Check sheet for the modelled part. Datum: model origin and axes. Units: mm. A direction names the side the tool comes from. Coordinates: 2 decimals unless noted, no trailing zeros. Write each loop counter-clockwise with the first axis right and the second up, starting at its lowest first coordinate (ties: lowest second). Pieces come first, ordered by that corner, then holes. Notation, with made-up numbers: (14, -25) -> (44, -25) arc R17 cw to (44, -21) -> close; hole circle Ø5 at (40, 38). An arc over 180 degrees is marked (long way). One line per item, written item: value. Start each with the question number.
1) Sectioned sample at D-D on x = -78. Enter the section's corners in (y, z), plus the area to 3 significant figures.
2) Sectioned sample at A-A on x = 0. Enter the section's corners in (y, z), plus the area to 3 significant figures.
3) Set-up check for faces 5 (the flat face through (29, -224, 7)), 6 (the flat face through (-82.516, -196.574, 3.451)): record each of +Z, -Z, +X, -X, +Y, -Y from which the full face is reachable in a straight line by a thin tool's end or side.
4) Gauge pin test, flat ends, axial feed: P1, Ø3, axis at x = -57, z = 4.5, coming from the -Y side; P2, Ø1.5, axis at x = 26.5, y = -417.5, coming from the -Z side; P3, Ø2, axis at x = -54.5, z = 4.5, coming from the +Y side; P4, Ø2, axis at x = -0.5, z = 1, coming from the -Y side. Record the tip position at first contact, or that the pin passes through.
5) Draft check along Y on faces 1 (the cylindrical face through (-178.984, -61.978, 3.451)), 2 (the flat face through (-100.6, 13.3, 3.5)), 3 (the cylindrical face through (-125.96, -269.94, 3.45)), 4 (the cylindrical face through (22.38, -43.028, 3.451)). Enter one of: +Y half, -Y half, draft (parallel to the pull), parting line (faces both ways), or undercut.
6) Sectioned sample at B-B on z = 5.75. Enter the section's corners in (x, y), plus the area to 3 significant figures.
7) Scan lines: line 1 along X through (y, z) = (-92, 2.25); line 2 along X through (y, z) = (-175, 4.75); line 3 along Y through (x, z) = (-134, 4). Record each from-to range of solid material in increasing order. Write a range as [from, to].
8) Sectioned sample at C-C on y = -117. Enter the section's corners in (x, z), plus the area to 3 significant figures.
```python
from build123d import *

# Parameters (mm, degrees)
SKETCH1_R      = 48.5
SKETCH1_R_2    = 46
EXTRUDE1_DEPTH = 7


with BuildPart() as part:
    # Sketch1 → Extrude1 (new body)
    with BuildSketch(Plane.XY):
        with BuildLine():
            Line((-181.296983893, -100.123158622), (-146.60541801, -252.204231237))
            ThreePointArc((-146.60541801, -252.204231237), (-125.550644715, -269.965422259), (-102.674010073, -254.621922903))
            Line((-102.674010073, -254.621922903), (-61.786520036, -136.878304089))
            ThreePointArc((-61.786520036, -136.878304089), (-17.984074435, -110.454979585), (15.979150749, -148.708680759))
            Line((15.979150749, -148.708680759), (22.803821631, -360))
            ThreePointArc((22.803821631, -360), (39.422409163, -464.1696592), (81.472905946, -560.912881546))
            Line((81.472905946, -560.912881546), (119.560838109, -625.042587939))
            ThreePointArc((119.560838109, -625.042587939), (124.22199896, -626.808768638), (126.985562325, -622.660451839))
            Line((126.985562325, -622.660451839), (122.910471509, -574.827683832))
            ThreePointArc((122.910471509, -574.827683832), (122.67212546, -573.014734487), (122.269195455, -571.231130949))
            Line((122.269195455, -571.231130949), (103.049494252, -501.215851748))
            ThreePointArc((103.049494252, -501.215851748), (90.834692996, -443.626181209), (85.473499156, -385))
            Line((85.473499156, -385), (72.961950117, 2.356657615))
            ThreePointArc((72.961950117, 2.356657615), (30.664556943, 66.247150486), (-45.416584246, 57.151849274))
            Line((-45.416584246, 57.151849274), (-157.305859298, -31.76266095))
            ThreePointArc((-157.305859298, -31.76266095), (-179.163336866, -62.481869477), (-181.296983893, -100.123158622))
        make_face()
        Circle(SKETCH1_R, mode=Mode.SUBTRACT)
        with Locations((-115, -85)):
            Circle(SKETCH1_R_2, mode=Mode.SUBTRACT)
    extrude(amount=EXTRUDE1_DEPTH)


solid = part.part
```
Answers:
1. outline: (-183.57, 0) -> (-112.33, 0) -> (-112.33, 7) -> (-183.57, 7) -> close; (-57.67, 0) -> (31.26, 0) -> (31.26, 7) -> (-57.67, 7) -> close
1. area: 1,120 mm2
2. outline: (-118, 0) -> (-48.5, 0) -> (-48.5, 7) -> (-118, 7) -> close; (48.5, 0) -> (73, 0) -> (73, 7) -> (48.5, 7) -> close
2. area: 658 mm2
3. face 5: +Z, +X, -X, +Y, -Y
3. face 6: +Z, -Z, -Y
4. P1: stops at y = -129.76
4. P2: passes through
4. P3: stops at y = 50.73
4. P4: stops at y = -118.38
5. face 1: parting line
5. face 2: +Y half
5. face 3: -Y half
5. face 4: undercut
6. outline: (-181.3, -100.12) -> (-146.61, -252.2) arc R22.89 ccw to (-102.67, -254.62) -> (-61.79, -136.88) arc R40 cw to (15.98, -148.71) -> (22.8, -360) arc R420 ccw to (81.47, -560.91) -> (119.56, -625.04) arc R4 ccw to (126.99, -622.66) -> (122.91, -574.83) arc R20 ccw to (122.27, -571.23) -> (103.05, -501.22) arc R500 cw to (85.47, -385) -> (72.96, 2.36) arc R73 ccw to (-45.42, 57.15) -> (-157.31, -31.76) arc R68 ccw to start; hole circle Ø92 at (-115, -85); hole circle Ø97 at (0, 0)
6. area: 62,800 mm2
7. line 1: x = [-182.64, -160.46], [-69.54, 76.01]
7. line 2: x = [-164.22, -75.02], [16.83, 78.69]
7. line 3: y = [-267.84, -126.89], [-43.11, -13.24]
8. outline: (-177.45, 0) -> (-148.05, 0) -> (-148.05, 7) -> (-177.45, 7) -> close; (-81.95, 0) -> (-46.61, 0) -> (-46.61, 7) -> (-81.95, 7) -> close; (-1.39, 0) -> (76.82, 0) -> (76.82, 7) -> (-1.39, 7) -> close
8. area: 1,000 mm2
